Verification items for the finished model (mm, model axes). A direction names the side the tool comes from. Round coordinates to 2 decimals unless told otherwise and drop trailing zeros. Order: outer loops, then holes, each group sorted by start corner. A loop starts at its lowest first (then second) coordinate and runs counter-clockwise, first axis right, second up. Notation, with made-up numbers: (60, -5) -> (92, -5) arc R14 ccw to (92, 6) -> close; hole circle Ø11 at (36, -31.5). An arc over 180 degrees is marked (long way). Return JSON: item names as keys, results as strings. Group by question number.
1) Depth check by flat-ended pin: pin 1 (4 mm diameter, centred on y = -15, z = 45, fed in from +X); pin 2 (12 mm diameter, centred on x = -17, y = -22, fed in from -Z). Enter the tip coordinate at first touch or a pass-through.
2) Scan lines: L1, parallel to Z at x = 13.5, y = -16.5; L2, parallel to Z at x = -21.95, y = 15; L3, parallel to Y at x = 0, z = 3. Record each from-to range of solid material in increasing order.
3) Section check A-A on x = 0. State how many separate pieces and enclosed holes the cut face has, plus the area to 3 significant figures.
4) Section check C-C on z = 32. Enter the section's corners in (x, y).
5) Draft check along X on faces 4 (the cylindrical face through (5.72, -1.1, 3.94)), 5 (the flat face through (-23, 0, 45)), 6 (the cylindrical face through (21.48, 15.07, 46.5)). Enter one of: pulls with the +X half, pulls with the -X half, needs draft (parallel to the pull), parting line crosses it, or undercut.
6) Section check D-D on y = -23. Enter the section's corners in (x, z), plus the area to 3 significant figures.
7) Section check B-B on z = 45. Enter the section's corners in (x, y), plus the area to 3 significant figures.
8) Tool access check on faces 1 (the cylindrical face through (-0.325, -16.464, 66.521)), 2 (the flat face through (3.2, -8.1, 10)), 3 (the flat face through (0, 0, 65)). Record the directions out of +Z, -Z, +X, -X, +Y, -Y that give a thin tool (end or side, any length) a straight path to the whole face; none if there is none.
```python
from build123d import *

# Parameters (mm, degrees)
ESQUISSE1_R                  = 8.5
BOSS_EXTRU_1_DEPTH           = 10
ESQUISSE2_R                  = 11
BOSS_EXTRU_2_DEPTH           = 12
ESQUISSE3_R                  = 2
ENL_V_MAT_EXTRU_1_DEPTH      = 8
CHANFREIN1_SIZE              = 1
BOSS_EXTRU_3_DEPTH           = 30
BOSS_EXTRU_3_DEPTH_BACK      = 30
ESQUISSE4_W                  = 46
ESQUISSE4_H                  = 46
ESQUISSE4_W_2                = 40
ESQUISSE4_H_2                = 40
ENL_V_MAT_EXTRU_2_DEPTH      = 88.407093534
ENL_V_MAT_EXTRU_2_DEPTH_BACK = 88.407093534
ESQUISSE5_R                  = 1.5
ESQUISSE6_R                  = 1.5
ENL_V_MAT_EXTRU_3_DEPTH      = 10
CONG_1_R                     = 10


with BuildPart() as part:
    # Esquisse1 → Boss.-Extru.1 (new body)
    with BuildSketch(Plane.XY):
        Circle(ESQUISSE1_R)
    extrude(amount=BOSS_EXTRU_1_DEPTH)

    # Esquisse2 → Boss.-Extru.2 (add)
    with BuildSketch(Plane.XY.offset(10)):
        Circle(ESQUISSE2_R)
    extrude(amount=BOSS_EXTRU_2_DEPTH)

    # Esquisse3 → Enlèv. mat.-Extru.1 (cut)
    with BuildSketch(Plane(origin=(0, 0, 0), x_dir=(-1, 0, 0), z_dir=(0, 0, -1))):
        with Locations((0, 4.9)):
            Circle(ESQUISSE3_R)
        with Locations((4.243524479, -2.45)):
            Circle(ESQUISSE3_R)
        with Locations((-4.243524479, -2.45)):
            Circle(ESQUISSE3_R)
    extrude(amount=-ENL_V_MAT_EXTRU_1_DEPTH, mode=Mode.SUBTRACT)

    # Chanfrein1
    chanfrein1_edges = [part.edges().sort_by_distance(p)[0] for p in [
        (-8.5, 0, 0),
    ]]
    chamfer(chanfrein1_edges, length=CHANFREIN1_SIZE)

    # Esquisse4 → Boss.-Extru.3 (add, two sides: drawn at the far end of the back side and taken through both)
    with BuildSketch(Plane(origin=(0, 0, 0), x_dir=(1, 0, 0), z_dir=(0, 1, 0)).offset(-BOSS_EXTRU_3_DEPTH_BACK)):
        with Locations((0, -45)):
            Rectangle(ESQUISSE4_W, ESQUISSE4_H)
        with Locations((0, -45)):
            Rectangle(ESQUISSE4_W_2, ESQUISSE4_H_2, mode=Mode.SUBTRACT)
    extrude(amount=BOSS_EXTRU_3_DEPTH + BOSS_EXTRU_3_DEPTH_BACK)

    # Esquisse5 → Enlèv. mat.-Extru.2 (cut, two sides: drawn at the far end of the back side and taken through both)
    with BuildSketch(Plane(origin=(23, 0, 0), x_dir=(0, 0, -1), z_dir=(1, 0, 0)).offset(-ENL_V_MAT_EXTRU_2_DEPTH_BACK)):
        with Locations((-45, 15)):
            Circle(ESQUISSE5_R)
        with Locations((-45, -15)):
            Circle(ESQUISSE5_R)
    extrude(amount=ENL_V_MAT_EXTRU_2_DEPTH + ENL_V_MAT_EXTRU_2_DEPTH_BACK, mode=Mode.SUBTRACT)

    # Esquisse6 → Enlèv. mat.-Extru.3 (cut)
    with BuildSketch(Plane.XY.offset(68)):
        with Locations((0, 15)):
            Circle(ESQUISSE6_R)
        with Locations((0, -15)):
            Circle(ESQUISSE6_R)
    extrude(amount=-ENL_V_MAT_EXTRU_3_DEPTH, mode=Mode.SUBTRACT)

    # Congé1
    cong_1_edges = [part.edges().sort_by_distance(p)[0] for p in [
        (-11, 0, 22),
    ]]
    fillet(cong_1_edges, radius=CONG_1_R)


solid = part.part
```
Check result:
{
 "1": {"pin 1": "x = 23", "pin 2": "z = 22"},
 "2": {"L1": "22 to 25, 65 to 68", "L2": "22 to 43.5, 46.5 to 68", "L3": "-8.5 to 2.9, 6.9 to 8.5"},
 "3": {"separate pieces": "4", "enclosed holes": "0", "area": "786 mm^2"},
 "4": {"outline": "(-23, -30) -> (-20, -30) -> (-20, 30) -> (-23, 30) -> close; (20, -30) -> (23, -30) -> (23, 30) -> (20, 30) -> close"},
 "5": {"face 4": "undercut", "face 5": "pulls with the -X half", "face 6": "needs draft"},
 "6": {"outline": "(-23, 22) -> (23, 22) -> (23, 68) -> (-23, 68) -> close; hole (-20, 25) -> (20, 25) -> (20, 65) -> (-20, 65) -> close", "area": "516 mm^2"},
 "7": {"outline": "(-23, -30) -> (-20, -30) -> (-20, -16.5) -> (-23, -16.5) -> close; (-23, -13.5) -> (-20, -13.5) -> (-20, 13.5) -> (-23, 13.5) -> close; (-23, 16.5) -> (-20, 16.5) -> (-20, 30) -> (-23, 30) -> close; (20, -30) -> (23, -30) -> (23, -16.5) -> (20, -16.5) -> close; (20, -13.5) -> (23, -13.5) -> (23, 13.5) -> (20, 13.5) -> close; (20, 16.5) -> (23, 16.5) -> (23, 30) -> (20, 30) -> close", "area": "324 mm^2"},
 "8": {"face 1": "+Z", "face 2": "-Z", "face 3": "+Y, -Y"}
}
